```python
from build123d import *

# Parameters (mm, degrees)
SKETCH_1_R          = 3
EXTRUDE_1_DEPTH     = 33
SKETCH_2_R          = 1.3
CUT_EXTRUDE_1_DEPTH = 5
CUT_EXTRUDE_START   = -5
SKETCH_3_R          = 1.3
CUT_EXTRUDE_2_DEPTH = 5
SKETCH_4_R          = 7.5
SKETCH_4_R_2        = 3
EXTRUDE_2_DEPTH     = 15


with BuildPart() as part:
    # ｽｹｯﾁ1 → ﾎﾞｽ - 押し出し1 (new body)
    with BuildSketch(Plane(origin=(0, 0, 0), x_dir=(0, 0, -1), z_dir=(1, 0, 0))):
        Circle(SKETCH_1_R)
    extrude(amount=EXTRUDE_1_DEPTH)

    # ｽｹｯﾁ2 → ｶｯﾄ - 押し出し1 (cut)
    with BuildSketch(Plane(origin=(33, 0, 0), x_dir=(0, 0, -1), z_dir=(1, 0, 0))):
        Circle(SKETCH_2_R)
    extrude(amount=-CUT_EXTRUDE_1_DEPTH, mode=Mode.SUBTRACT)

    # ｽｹｯﾁ3 → ｶｯﾄ - 押し出し2 (cut)
    with BuildSketch(Plane.ZY.offset(CUT_EXTRUDE_START)):
        with Locations(Location((0, 0, 0), (0, 0, 180))):
            Circle(SKETCH_3_R)
    extrude(amount=CUT_EXTRUDE_2_DEPTH, mode=Mode.SUBTRACT)

    # ｽｹｯﾁ4 → ﾎﾞｽ - 押し出し2 (add)
    with BuildSketch(Plane(origin=(0, 0, 0), x_dir=(0, 0, -1), z_dir=(1, 0, 0))):
        Circle(SKETCH_4_R)
        Circle(SKETCH_4_R_2, mode=Mode.SUBTRACT)
    extrude(amount=EXTRUDE_2_DEPTH)


solid = part.part
```
Check sheet for the modelled part. Datum: model origin and axes. Units: mm. A direction names the side the tool comes from. Coordinates: 2 decimals unless noted, no trailing zeros. Write each loop counter-clockwise with the first axis right and the second up, starting at its lowest first coordinate (ties: lowest second). Pieces come first, ordered by that corner, then holes. Notation, with made-up numbers: M 55.5,72 L 73.5,72 A32 ccw 73.5,101 Z; hole C 39.25,-27 d2. An arc over 180 degrees is marked long. Use one line per item in the form item = value.
Item 1: Sectioned sample at D-D, the plane y = 2.5. Record the cut outline in (x, z), and give its area (3 significant figures).
Answer below:
outline = M 0,-7.07 L 15,-7.07 L 15,-1.66 L 33,-1.66 L 33,1.66 L 15,1.66 L 15,7.07 L 0,7.07 Z
area = 272 mm^2
Item 2: Gauge pin test, flat ends, axial feed: pin 1 Ø2 at (y, z) = (-5.5, -1) entering from +X; pin 2 Ø3 at (x, y) = (11, 4) entering from +Z; pin 3 Ø3 at (y, z) = (0, 0) entering from +X; pin 4 Ø1.5 at (x, y) = (22, -3.5) entering from +Z. Record the tip position at first contact, or that the pin passes through.
Answer below:
pin_1 = 15
pin_2 = 7.07
pin_3 = 33
pin_4 = 1.2
Item 3: Release check for a two-part mould opening along Z. For faces 4 (the face through (5, 0, 0)), 5 (the face through (24, 0, 3)), 6 (the face through (0, 0, -2)) record: pulls with the +Z half, pulls with the -Z half, needs draft (parallel to the pull), parting line crosses it, or undercut.
Answer below:
face_4 = undercut
face_5 = parting line crosses it
face_6 = needs draft
Item 4: Sectioned sample at C-C, the plane z = 2. Record the cut outline in (x, y).
Answer below:
outline = M 0,-7.23 L 15,-7.23 L 15,-2.24 L 33,-2.24 L 33,2.24 L 15,2.24 L 15,7.23 L 0,7.23 Z
Item 5: Material ranges on L1, parallel to Y at x = 1.15, z = 0; L2, parallel to Y at x = 29.8, z = 0; L3, parallel to X at y = 5.75, z = -2.5, recorded low to high. Write a range as from..to.
Answer below:
L1 = -7.5..-1.3, 1.3..7.5
L2 = -3..-1.3, 1.3..3
L3 = 0..15
Item 6: Sectioned sample at A-A, the plane z = 0. Record the cut outline in (x, y).
Answer below:
outline = M 0,-7.5 L 15,-7.5 L 15,-3 L 33,-3 L 33,-1.3 L 28,-1.3 L 28,1.3 L 33,1.3 L 33,3 L 15,3 L 15,7.5 L 0,7.5 L 0,1.3 L 5,1.3 L 5,-1.3 L 0,-1.3 Z
Item 7: Set-up check for faces 1 (the face through (2.54, -0.39, -1.24)), 2 (the face through (7.395, 0.33, 7.493)), 3 (the face through (28, 0, 0)): record each of +Z, -Z, +X, -X, +Y, -Y from which the full face is reachable in a straight line by a thin tool's end or side.
Answer below:
face_1 = -X
face_2 = +X, -X
face_3 = +X
